Input: dimensioned drawing with shaded views. Units: mm. Origin: part minimum x, y, z. A direction names the side the tool comes from. Round coordinates to 2 decimals unless told otherwise and drop trailing zeros. Write each loop counter-clockwise with the first axis right and the second up, starting at its lowest first coordinate (ties: lowest second). Pieces come first, ordered by that corner, then holes. Notation, with made-up numbers: (-38, -12.5) -> (10, -12.5) arc R25 cw to (10, 25.5) -> close; hole circle Ø7 at (-19.5, 32). An arc over 180 degrees is marked (long way). Return JSON: item names as keys, results as strings. Group by question number.
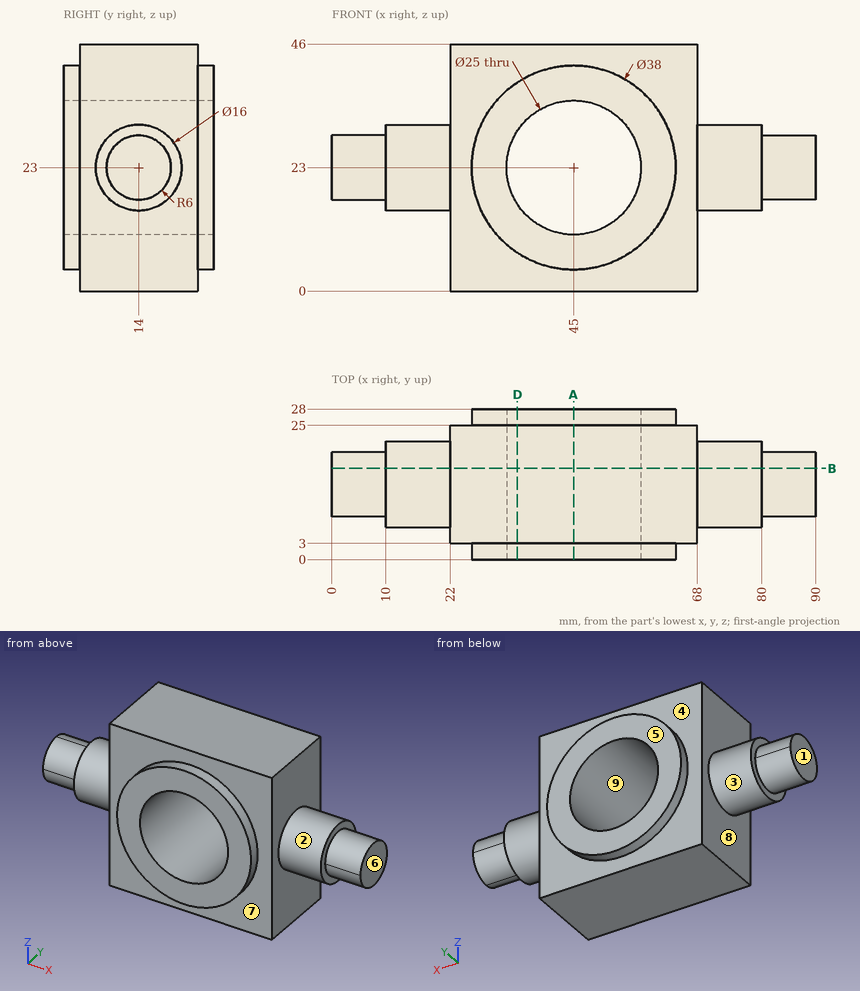
Item 1: Cut plane B-B on y = 17. Output: boundary loops of the cut face in (x, z).
Item 2: Material intervals for probe 1 along X at (y, z) = (21, 23); probe 2 along X at (y, z) = (14, 23); probe 3 along Y at (x, z) = (67.5, 14.5), sorted ascending.
Item 3: Set-up query: the marked faces 1, 2, 3, 4 and 5. Return all of +Z, -Z, +X, -X, +Y, -Y with unobstructed straight access to the full face (end or side cutting, diameter ignored); none if empty.
Item 4: Cut plane A-A on x = 45. Output: boundary loops of the cut face in (y, z).
Item 5: Cut plane D-D on x = 34.5. Output: boundary loops of the cut face in (y, z).
Item 6: Pull-direction query (X, two-part tool) for the marked faces 6, 7, 8 and 9; classes: +X half, -X half, draft (parallel to the pull), parting line (faces both ways), or undercut.
Item 7: First-contact query: pin 1 Ø1.5 at (x, z) = (13, 26) entering from -Y; pin 2 Ø3 at (x, z) = (23, 34) entering from +Y; pin 3 Ø1 at (y, z) = (19, 36) entering from -X. Flat tips, straight axial feed; report the tip coordinate or a pass-through.
Here are the results:
{
 "1": {"outline": "(0, 17.8) -> (10, 17.8) -> (10, 15.58) -> (22, 15.58) -> (22, 0) -> (68, 0) -> (68, 15.58) -> (80, 15.58) -> (80, 17.8) -> (90, 17.8) -> (90, 28.2) -> (80, 28.2) -> (80, 30.42) -> (68, 30.42) -> (68, 46) -> (22, 46) -> (22, 30.42) -> (10, 30.42) -> (10, 28.2) -> (0, 28.2) -> close; hole circle Ø25 at (45, 23)"},
 "2": {"probe 1": "x = 10 to 32.5, 57.5 to 80", "probe 2": "x = 0 to 32.5, 57.5 to 90", "probe 3": "y = 3 to 25"},
 "3": {"face 1": "+Z, -Z, -X, +Y, -Y", "face 2": "+X", "face 3": "-X", "face 4": "+Y", "face 5": "+Z, -Z, +X, -X, +Y"},
 "4": {"outline": "(0, 4) -> (3, 4) -> (3, 0) -> (25, 0) -> (25, 4) -> (28, 4) -> (28, 10.5) -> (0, 10.5) -> close; (0, 35.5) -> (28, 35.5) -> (28, 42) -> (25, 42) -> (25, 46) -> (3, 46) -> (3, 42) -> (0, 42) -> close"},
 "5": {"outline": "(0, 7.16) -> (3, 7.16) -> (3, 0) -> (25, 0) -> (25, 7.16) -> (28, 7.16) -> (28, 16.22) -> (0, 16.22) -> close; (0, 29.78) -> (28, 29.78) -> (28, 38.84) -> (25, 38.84) -> (25, 46) -> (3, 46) -> (3, 38.84) -> (0, 38.84) -> close"},
 "6": {"face 6": "+X half", "face 7": "draft", "face 8": "-X half", "face 9": "undercut"},
 "7": {"pin 1": "stops at y = 6.32", "pin 2": "stops at y = 25", "pin 3": "stops at x = 22"}
}
